Input: part model. Units: mm. Frame: model coordinates. Face numbers are marked on the shaded views. Give positions to 0.01 mm unless a question says otherwise; leave off trailing zeros. Loops run counter-clockwise (first coordinate to the right, second up) from the corner with the lowest first, then second, coordinate; pieces in that order, holes last.
from build123d import *

# Parameters (mm, degrees)
BOSS_EXTRUDE2_DEPTH = 160
CUT_EXTRUDE1_DEPTH  = 150
SKETCH3_R           = 7.5
CUT_EXTRUDE2_DEPTH  = 10


with BuildPart() as part:
    # Sketch1 → Boss-Extrude2 (new body)
    with BuildSketch(Plane(origin=(0, 0, 0), x_dir=(1, 0, 0), z_dir=(0, 1, 0))):
        with BuildLine():
            Line((-40, 80), (40, 80))
            Line((40, 80), (40, 91.651513899))
            ThreePointArc((40, 91.651513899), (0, -100), (-40, 91.651513899))
            Line((-40, 91.651513899), (-40, 80))
        make_face()
    extrude(amount=-BOSS_EXTRUDE2_DEPTH)

    # Sketch2 → Cut-Extrude1 (cut)
    with BuildSketch(Plane(origin=(0, 0, 0), x_dir=(1, 0, 0), z_dir=(0, 1, 0))):
        with BuildLine():
            Line((-50, 74.833147735), (-50, 70))
            Line((-50, 70), (50, 70))
            Line((50, 70), (50, 74.833147735))
            ThreePointArc((50, 74.833147735), (0, -90), (-50, 74.833147735))
        make_face()
    extrude(amount=-CUT_EXTRUDE1_DEPTH, mode=Mode.SUBTRACT)

    # Sketch3 → Cut-Extrude2 (cut)
    with BuildSketch(Plane(origin=(0, 0, -80), x_dir=(-1, 0, 0), z_dir=(0, 0, -1))):
        with Locations(Location((0, -120, 0), (0, 0, 180))):
            Circle(SKETCH3_R)
    extrude(amount=-CUT_EXTRUDE2_DEPTH, mode=Mode.SUBTRACT)


solid = part.part
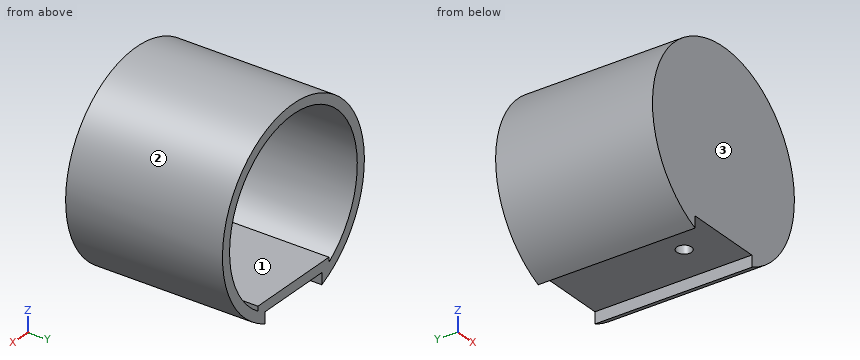
(1) Pin query (flat end, axial travel): pin 1 Ø2 at (y, z) = (-84, 63) entering from +X; pin 2 Ø1.5 at (x, y) = (72.5, -127.5) entering from +Z; pin 3 Ø13 at (y, z) = (-75.5, -83.5) entering from -X. Return the tip coordinate at first contact, or that it passes through.
Values follow:
pin 1: stops at x = 78.46
pin 2: stops at z = 69.66
pin 3: stops at x = -63.8
(2) Ray query, probe 1 along Y at (x, z) = (0, -73); probe 2 along X at (y, z) = (-120, -72); probe 3 along Z at (x, y) = (0, -55). Return the intervals inside material, ascending.
Values follow:
probe 1: y = -160 to -127.5, -112.5 to 0
probe 2: x = -69.4 to -54, -50 to -7.5, 7.5 to 50, 54 to 69.4
probe 3: z = -80 to -70, 90 to 100
(3) Cut plane B-B (y = -120). Return the cut outline in (x, z).
Values follow:
outline: (-50, -74.83) arc R90 cw (long way) to (50, -74.83) - (50, -70) - (7.5, -70) - (7.5, -80) - (40, -80) - (40, -91.65) arc R100 ccw (long way) to (-40, -91.65) - (-40, -80) - (-7.5, -80) - (-7.5, -70) - (-50, -70) - close
(4) Cut plane C-C (y = -14.5). Return the cut outline in (x, z).
Values follow:
outline: (-40, -91.65) - (-40, -80) - (40, -80) - (40, -91.65) arc R100 ccw (long way) to start; hole (-50, -74.83) - (-50, -70) - (50, -70) - (50, -74.83) arc R90 ccw (long way) to start
(5) Cut plane A-A (x = 0). Return the cut outline in (y, z).
Values follow:
outline: (-160, -80) - (-127.5, -80) - (-127.5, -70) - (-150, -70) - (-150, 90) - (0, 90) - (0, 100) - (-160, 100) - close; (-112.5, -80) - (0, -80) - (0, -70) - (-112.5, -70) - close
(6) Cut plane D-D (z = -3). Return the cut outline in (x, y), and give its area (3 significant figures).
Values follow:
outline: (-99.95, -160) - (99.95, -160) - (99.95, 0) - (89.95, 0) - (89.95, -150) - (-89.95, -150) - (-89.95, 0) - (-99.95, 0) - close
area: 5,000 mm2
(7) Mould query, pull axis X, two halves, no side actions, for the marked faces 1, 2 and 3. Classes: +X half, -X half, draft (parallel to the pull), parting line (faces both ways), or undercut.
Values follow:
face 1: undercut
face 2: parting line
face 3: draft
